```python
from build123d import *

# Parameters (mm, degrees)
BOSS_EXTRUDE1_DEPTH = 10
BOSS_EXTRUDE2_DEPTH = 10
FILLET2_R           = 0.5
CUT_EXTRUDE1_DEPTH  = 7


with BuildPart() as part:
    # Sketch1 → Boss-Extrude1 (new body)
    with BuildSketch(Plane(origin=(0, 0, 0), x_dir=(1, 0, 0), z_dir=(0, 1, 0))):
        Polygon((4.145480081, 4.393952182), (3.02042302, 5.231526131), (1.732534173, 5.787067152), (0.351243959, 6.030625884), (-1.048981906, 5.949072015), (-2.392656886, 5.546802133), (-3.607343114, 4.845502712), (-4.627556541, 3.882980986), (-5.398297196, 2.71112675), (-5.878014253, 1.39311497), (-6.04084604, 0), (-5.878014253, -1.39311497), (-5.398297196, -2.71112675), (-4.627556541, -3.882980986), (-3.607343114, -4.845502712), (-2.392656886, -5.546802133), (-1.048981906, -5.949072015), (0.351243959, -6.030625884), (1.732534173, -5.787067152), (3.02042302, -5.231526131), (4.145480081, -4.393952182), (5.047053237, -3.319499134), (5.676538447, -2.066091028), (6, -0.701299421), (6, 0.701299421), (5.676538447, 2.066091028), (5.047053237, 3.319499134), align=None)
    extrude(amount=BOSS_EXTRUDE1_DEPTH)

    # Sketch2 → Boss-Extrude2 (add)
    with BuildSketch(Plane(origin=(0, 0, 0), x_dir=(1, 0, 0), z_dir=(0, 1, 0))):
        Polygon((-1.094764488, 6.735128586), (0.305461378, 6.816682456), (0.351243959, 6.030625884), (-1.048981906, 5.949072015), align=None)
    extrude(amount=BOSS_EXTRUDE2_DEPTH)

    # Fillet2
    fillet2_edges = [part.edges().sort_by_distance(p)[0] for p in [
        (4.596266659, 10, 3.856725658),
        (5.361795842, 10, 2.692795081),
        (5.838269223, 10, 1.383695224),
        (5.361795842, 10, -2.692795081),
        (4.596266659, 10, -3.856725658),
        (3.58295155, 10, -4.812739157),
        (2.376478596, 10, -5.509296641),
        (1.041889066, 10, -5.908846518),
        (-1.720819396, 10, -5.747937074),
        (-3, 10, -5.196152423),
        (-4.117449827, 10, -4.364241849),
        (-5.012926868, 10, -3.297053868),
        (6, 10, 0),
        (-5.638155725, 10, -2.05212086),
        (-5.959430146, 10, -0.696557485),
        (-5.959430146, 10, 0.696557485),
        (-5.638155725, 10, 2.05212086),
        (-5.012926868, 10, 3.297053868),
        (-4.117449827, 10, 4.364241849),
        (-3, 10, 5.196152423),
        (-1.720819396, 10, 5.747937074),
        (-0.348868973, 10, 5.98984895),
        (1.041889066, 10, 5.908846518),
        (5.838269223, 10, -1.383695224),
        (2.376478596, 10, 5.509296641),
        (3.58295155, 10, 4.812739157),
    ]]
    fillet(fillet2_edges, radius=FILLET2_R)

    # Sketch4 → Cut-Extrude1 (cut)
    with BuildSketch(Plane(origin=(0, 0, 0), x_dir=(1, 0, 0), z_dir=(0, 1, 0))):
        with BuildLine():
            ThreePointArc((3.45, 0), (2.439518395, 2.439518395), (0, 3.45))
            Line((0, 3.45), (0, -1.55))
            Line((0, -1.55), (3.082207001, -1.55))
            ThreePointArc((3.082207001, -1.55), (3.356792677, -0.796519254), (3.45, 0))
        make_face()
        with BuildLine():
            Line((0, -1.55), (0, 3.45))
            ThreePointArc((0, 3.45), (-2.936835031, 1.810386699), (-3.082207001, -1.55))
            Line((-3.082207001, -1.55), (0, -1.55))
        make_face()
    extrude(amount=CUT_EXTRUDE1_DEPTH, mode=Mode.SUBTRACT)


solid = part.part
```
For this review, take the finished solid that the model builds, in its own axes (mm). Coordinates: 2 decimals unless noted, no trailing zeros. Return JSON: item names as keys, results as strings. Group by question number.
(1) Mouldability with a two-part tool opening along X and no side actions: class faces 1 (the cylindrical face through (3.501, 9.857, 4.686)), 2 (the cylindrical face through (-2.93, 9.86, -5.06)), 3 (the flat face through (0, 3, 1.55)), 4 (the flat face through (0, 7, 0)) as pulls with the +X half, pulls with the -X half, needs draft (parallel to the pull), parting line crosses it, or undercut.
(2) For pin 1 Ø6 at (y, z) = (3.5, -3.5) entering from -X; pin 2 Ø4 at (y, z) = (6.5, -5) entering from +X; pin 3 Ø5 at (y, z) = (1.5, 3.5) entering from -X, all flat-tipped, find the tip position at first contact; note any pin that passes through.
(3) To check wall thickness, follow L1, parallel to Y at x = 0.5, z = -0.25; L2, parallel to X at y = 3, z = -2; L3, parallel to X at y = 1, z = -1.75. State the ranges of each line that lie inside material, in increasing order.
Results below:
{
 "1": {"face 1": "pulls with the +X half", "face 2": "pulls with the -X half", "face 3": "undercut", "face 4": "undercut"},
 "2": {"pin 1": "stops at x = -5.98", "pin 2": "stops at x = 5.21", "pin 3": "stops at x = -5.92"},
 "3": {"L1": "y = 7 to 10", "L2": "x = -5.66 to -2.81, 2.81 to 5.69", "L3": "x = -5.75 to -2.97, 2.97 to 5.75"}
}
